Design review of the part built by this model. Coordinates are the model's own, in mm. Give positions to 0.01 mm unless a question says otherwise; leave off trailing zeros. Write each loop counter-clockwise with the first axis right and the second up, starting at its lowest first coordinate (ties: lowest second). Pieces come first, ordered by that corner, then holes. Notation, with made-up numbers: M -23.5,4 L -2.5,4 A30 ccw -2.5,35 Z; hole C 82,80.25 d8. An arc over 180 degrees is marked long. Use a Markdown table: item, result. Add a question column.
```python
from build123d import *

# Parameters (mm, degrees)
F0_R     = 11.162789
F0_R_2   = 10.9982
F1_DEPTH = 8.89


with BuildPart() as f1:
    # F0 (on Top) → F1 (new body)
    with BuildSketch(Plane.XY):
        with BuildLine():
            ThreePointArc((20.78403, 10.17702), (12.955474, 14.150564), (12.376799, 22.910729))
            ThreePointArc((12.376799, 22.910729), (0.831126, 51.33837), (-13.448812, 24.181111))
            ThreePointArc((-13.448812, 24.181111), (-13.323241, 15.251649), (-20.671656, 10.17702))
            ThreePointArc((-20.671656, 10.17702), (-21.084916, 0.863796), (-26.915357, -6.410328))
            ThreePointArc((-26.915357, -6.410328), (-35.876376, -36.540667), (-8.662071, -20.807938))
            ThreePointArc((-8.662071, -20.807938), (-4.331036, -17.634318), (0, -20.807938))
            ThreePointArc((0, -20.807938), (4.421541, -17.66469), (8.622223, -21.097517))
            ThreePointArc((8.622223, -21.097517), (37.152681, -35.425851), (23.821326, -6.416143))
            ThreePointArc((23.821326, -6.416143), (19.777657, 1.418246), (20.78403, 10.17702))
        make_face()
        with Locations((-25.4, -23.25872)):
            Circle(F0_R, mode=Mode.SUBTRACT)
        Circle(F0_R_2, mode=Mode.SUBTRACT)
        with Locations((25.4, -23.25872)):
            Circle(F0_R_2, mode=Mode.SUBTRACT)
        with Locations((0, 34.4424)):
            Circle(F0_R_2, mode=Mode.SUBTRACT)
    extrude(amount=F1_DEPTH)


solid = f1.part
```
(1) Add section A-A on x = 25.4. Give the boundary of the cut face in (y, z), then the cut area to 3 significant figures.
(2) The part is to be moulded in two halves that separate along Y. For faces 1 (the flat face through (3, -11, 8.89)), 2 (the cylindrical face through (19.8, 1.3, 4.4)), say which applies: released by +Y, released by -Y, zero draft, split by the parting line, or undercut.
(3) Add section B-B on y = 31.5. Give the boundary of the cut face in (x, z), then the cut area to 3 significant figures.
(4) Add section C-C on x = -4. Give the boundary of the cut face in (y, z), then the cut area to 3 significant figures.
(5) Wall thickness on L1, parallel to Y at x = 25.4, z = 3.75; L2, parallel to X at y = -14, z = 7; L3, parallel to Y at x = 15.5, z = 3.5: over which ranges is each line inside the solid? List them lowest first.
(6) For pin 1 (12 mm diameter, centred on x = 27.5, y = 27.5, fed in from +Z); pin 2 (4 mm diameter, centred on y = 6, z = 2, fed in from -X); pin 3 (4 mm diameter, centred on x = 28, z = 7, fed in from -Y); pin 4 (3 mm diameter, centred on y = 8, z = 4, fed in from +X), all flat-tipped, find the tip position at first contact; note any pin that passes through.
(7) Add section D-D on z = 3.5. Give the boundary of the cut face in (x, y), then the cut area to 3 significant figures.
From the geometry:
| question | item | result |
|---|---|---|
| 1 | outline | M -40.18,0 L -34.26,0 L -34.26,8.89 L -40.18,8.89 Z; M -12.26,0 L -6.34,0 L -6.34,8.89 L -12.26,8.89 Z |
| 1 | area | 105 mm^2 |
| 2 | face 1 | zero draft |
| 2 | face 2 | undercut |
| 3 | outline | M -16.66,0 L -10.6,0 L -10.6,8.89 L -16.66,8.89 Z; M 10.6,0 L 16.66,0 L 16.66,8.89 L 10.6,8.89 Z |
| 3 | area | 108 mm^2 |
| 4 | outline | M -17.65,0 L -10.25,0 L -10.25,8.89 L -17.65,8.89 Z; M 10.25,0 L 24.2,0 L 24.2,8.89 L 10.25,8.89 Z; M 44.69,0 L 50.88,0 L 50.88,8.89 L 44.69,8.89 Z |
| 4 | area | 245 mm^2 |
| 5 | L1 | y = -40.18 to -34.26, -12.26 to -6.34 |
| 5 | L2 | x = -39.56 to -31.64, -19.16 to 19.46, 31.34 to 39.56 |
| 5 | L3 | y = -36.98 to -28.05, -18.47 to 11.62, 27.67 to 41.22 |
| 6 | pin 1 | passes through |
| 6 | pin 2 | stops at x = -20.28 |
| 6 | pin 3 | stops at y = -40.16 |
| 6 | pin 4 | stops at x = 20.51 |
| 7 | outline | M -26.92,-6.41 A16.92 ccw long -8.66,-20.81 A4.54 cw 0,-20.81 A4.47 cw 8.62,-21.1 A16.92 ccw long 23.82,-6.42 A15.14 cw 20.78,10.18 A8.87 cw 12.38,22.91 A16.92 ccw long -13.45,24.18 A9.48 cw -20.67,10.18 A15.01 cw Z; hole C -25.4,-23.26 d22.33; hole C 0,0 d22; hole C 0,34.44 d22; hole C 25.4,-23.26 d22 |
| 7 | area | 2,440 mm^2 |
